Geometry: final body of the model. Coordinates: model frame, mm. A direction names the side the tool comes from. Give positions to 0.01 mm unless a question says otherwise; leave off trailing zeros. Order: outer loops, then holes, each group sorted by start corner. A loop starts at its lowest first (then second) coordinate and runs counter-clockwise, first axis right, second up. Notation, with made-up numbers: (69, -1) - (113, -1) arc R22 cw to (113, 26) - close; hole circle Ø1 at (78.5, -34). An arc over 180 degrees is marked (long way). Write item = value, one per line. Start each with the question number.
from build123d import *

# Parameters (mm, degrees)
SKETCH1_R           = 89
BOSS_EXTRUDE1_DEPTH = 90
CUT_EXTRUDE1_DEPTH  = 91
SKETCH3_R           = 80
CUT_EXTRUDE2_DEPTH  = 70
SKETCH4_R           = 10
CUT_EXTRUDE3_DEPTH  = 91


with BuildPart() as part:
    # Sketch1 → Boss-Extrude1 (new body)
    with BuildSketch(Plane.XY):
        with Locations((232.735026919, 15)):
            Circle(SKETCH1_R)
    extrude(amount=-BOSS_EXTRUDE1_DEPTH)

    # Sketch2 → Cut-Extrude1 (cut, through all)
    with BuildSketch(Plane.XY):
        with BuildLine():
            Line((221.301935747, 89.123440464), (230.448408684, 29.824688093))
            ThreePointArc((230.448408684, 29.824688093), (225.235026919, 27.990381057), (221.039779545, 24.392613526))
            Line((221.039779545, 24.392613526), (174.258790047, 61.963067631))
            ThreePointArc((174.258790047, 61.963067631), (195.235026919, 79.951905284), (221.301935747, 89.123440464))
        make_face()
        with BuildLine():
            Line((244.168118091, 89.123440464), (235.021645153, 29.824688093))
            ThreePointArc((235.021645153, 29.824688093), (240.235026919, 27.990381057), (244.430274293, 24.392613526))
            Line((244.430274293, 24.392613526), (291.211263791, 61.963067631))
            ThreePointArc((291.211263791, 61.963067631), (270.235026919, 79.951905284), (244.168118091, 89.123440464))
        make_face()
        with BuildLine():
            Line((162.825698875, 42.160372833), (218.75316131, 20.432074567))
            ThreePointArc((218.75316131, 20.432074567), (217.735026919, 15), (218.75316131, 9.567925433))
            Line((218.75316131, 9.567925433), (162.825698875, -12.160372833))
            ThreePointArc((162.825698875, -12.160372833), (157.735026919, 15), (162.825698875, 42.160372833))
        make_face()
        with BuildLine():
            Line((174.258790047, -31.963067631), (221.039779545, 5.607386474))
            ThreePointArc((221.039779545, 5.607386474), (225.235026919, 2.009618943), (230.448408684, 0.175311907))
            Line((230.448408684, 0.175311907), (221.301935747, -59.123440464))
            ThreePointArc((221.301935747, -59.123440464), (195.235026919, -49.951905284), (174.258790047, -31.963067631))
        make_face()
        with BuildLine():
            Line((244.168118091, -59.123440464), (235.021645153, 0.175311907))
            ThreePointArc((235.021645153, 0.175311907), (240.235026919, 2.009618943), (244.430274293, 5.607386474))
            Line((244.430274293, 5.607386474), (291.211263791, -31.963067631))
            ThreePointArc((291.211263791, -31.963067631), (270.235026919, -49.951905284), (244.168118091, -59.123440464))
        make_face()
        with BuildLine():
            Line((302.644354963, -12.160372833), (246.716892528, 9.567925433))
            ThreePointArc((246.716892528, 9.567925433), (247.735026919, 15), (246.716892528, 20.432074567))
            Line((246.716892528, 20.432074567), (302.644354963, 42.160372833))
            ThreePointArc((302.644354963, 42.160372833), (307.735026919, 15), (302.644354963, -12.160372833))
        make_face()
    extrude(amount=-CUT_EXTRUDE1_DEPTH, mode=Mode.SUBTRACT)

    # Sketch3 → Cut-Extrude2 (cut)
    with BuildSketch(Plane.XY):
        with Locations((232.735026919, 15)):
            Circle(SKETCH3_R)
    extrude(amount=-CUT_EXTRUDE2_DEPTH, mode=Mode.SUBTRACT)

    # Sketch4 → Cut-Extrude3 (cut, through all)
    with BuildSketch(Plane(origin=(0, 0, -90), x_dir=(-1, 0, 0), z_dir=(0, 0, -1))):
        with Locations((-232.735026919, 15)):
            Circle(SKETCH4_R)
    extrude(amount=-CUT_EXTRUDE3_DEPTH, mode=Mode.SUBTRACT)


solid = part.part
Q1. Section C-C, the plane z = -49. Return the cut outline in (x, y), then the cut area to 3 significant figures.
Q2. Section B-B, the plane x = 277. Return the cut outline in (y, z).
Q3. Section A-A, the plane y = 15. Return the cut outline in (x, z).
Q4. Contact query for flat-ended pins moving along their axis: pin 1 (1 mm diameter, centred on x = 215, z = -59.5, fed in from -Y); pin 2 (4 mm diameter, centred on x = 297, z = -11, fed in from +Y); pin 3 (5 mm diameter, centred on x = 300.5, z = -44.5, fed in from +Y). Output: stop coordinate, or through.
Q5. Pull-direction query (X, two-part tool) for faces 1 (the flat face through (159.8, 48.4, 0)), 2 (the cylindrical face through (143.82, 18.91, -44.37)), 3 (the cylindrical face through (223.498, 11.17, -80.14)); classes: +X half, -X half, draft (parallel to the pull), parting line (faces both ways), or undercut.
Q6. Material intervals for line 1 along X through (y, z) = (11, -83.5); line 2 along Y through (x, z) = (208.5, -75.5); line 3 along Y through (x, z) = (234, -44), sorted ascending. Write a range as from..to.
Q7. Set-up query: faces 4 (the cylindrical face through (194.899, 79.756, -79.86)), 5 (the cylindrical face through (152.812, 18.517, -34.51)). Return all of +Z, -Z, +X, -X, +Y, -Y with unobstructed straight access to the full face (end or side cutting, diameter ignored); none if empty.
The answers:
q1.outline = circle Ø178 at (232.74, 15); hole circle Ø160 at (232.74, 15)
q1.area = 4,780 mm²
q2.outline = (-62.21, -90) - (-45.54, -90) - (-45.54, -70) - (-51.64, -70) - (-51.64, 0) - (-62.21, 0) - close; (-20.55, -90) - (-2.2, -90) - (-2.2, -70) - (-20.55, -70) - close; (32.2, -90) - (50.55, -90) - (50.55, -70) - (32.2, -70) - close; (75.54, -90) - (92.21, -90) - (92.21, 0) - (81.64, 0) - (81.64, -70) - (75.54, -70) - close
q3.outline = (143.74, -90) - (157.74, -90) - (157.74, -70) - (152.74, -70) - (152.74, 0) - (143.74, 0) - close; (217.74, -90) - (222.74, -90) - (222.74, -70) - (217.74, -70) - close; (242.74, -90) - (247.74, -90) - (247.74, -70) - (242.74, -70) - close; (307.74, -90) - (321.74, -90) - (321.74, 0) - (312.74, 0) - (312.74, -70) - (307.74, -70) - close
q4.pin_1 = -72.32
q4.pin_2 = 78.59
q4.pin_3 = 75.51
q5.face_1 = draft
q5.face_2 = parting line
q5.face_3 = undercut
q6.line_1 = 143.82..157.84, 218.28..223.57, 241.9..247.19, 307.63..321.65
q6.line_2 = -70.64..-55.98, -4.46..5.58, 24.42..34.46, 85.98..100.64
q6.line_3 = -73.99..-64.99, 94.99..103.99
q7.face_4 = +Z, -Z
q7.face_5 = +Z
